Geometry: final body of the model. Coordinates: model frame, mm. A direction names the side the tool comes from. Give positions to 0.01 mm unless a question says otherwise; leave off trailing zeros. Loops run counter-clockwise (first coordinate to the right, second up) from the corner with the lowest first, then second, coordinate; pieces in that order, holes last. Notation, with made-up numbers: (8, 69.5) -> (41, 69.5) arc R15 cw to (41, 87.5) -> close; hole circle Ø6 at (19, 22). An arc over 180 degrees is marked (long way). Answer in a Markdown table with one row per item. Add a question column.
1) Section query A-A (y = -94). Return the cut outline in (x, z).
2) Line query: line 1 (Z direction, x = 0, y = -94); line 2 (Z direction, x = -99, y = -87); line 3 (X direction, y = -91, z = -73). Output: solid intervals per line, ascending. Write a range as from..to.
3) Section query D-D (z = -137). Return the cut outline in (x, y), plus the area to 3 significant figures.
4) First-contact query: P1, Ø2, axis at x = -19, z = -56, coming from the -Y side. Flat tip, straight axial feed; report the tip coordinate or a pass-through.
5) Section query C-C (z = 38.1). Return the cut outline in (x, y).
6) Draft query along X for faces 1 (the flat face through (-127, -60, -3)), 2 (the flat face through (-116.84, -68, -3)), 3 (the flat face through (-2, 0, -40)). Return one class per face: +X half, -X half, draft (parallel to the pull), parting line (faces both ways), or undercut.
7) Section query B-B (x = 0). Return the cut outline in (y, z), plus the area to 3 significant figures.
8) Access query for faces 4 (the flat face through (21.5, -127, 98.5)), 5 (the flat face through (-2, -68, -180.34)). Directions: +Z, -Z, +X, -X, +Y, -Y. A direction counts if a zero-diameter tool reaches every point of the face in a straight line with its end or side. Return the directions, or none.
```python
from build123d import *

# Parameters (mm, degrees)
F0_W     = 254
F0_H     = 381
F1_DEPTH = 127
F2_R     = 63.5
F3_DEPTH = 127.001
F4_T     = -10.16
F5_R     = 5.08


with BuildPart() as f1:
    # F0 (on Front) → F1 (new body)
    with BuildSketch(Plane.XZ):
        Rectangle(F0_W, F0_H)
    extrude(amount=F1_DEPTH)

    # F2 (on face) → F3 (cut, through all)
    with BuildSketch(Plane.XZ.offset(127)):
        with Locations((0, 38.1)):
            Circle(F2_R)
    extrude(amount=-F3_DEPTH, mode=Mode.SUBTRACT)

    # F4
    f4_openings = [f1.faces().sort_by_distance(p)[0] for p in [
        (0, -127, -185.92095),
    ]]
    offset(amount=F4_T, openings=f4_openings)

    # F5
    f5_edges = [f1.edges().sort_by_distance(p)[0] for p in [
        (-127, -127, 0),
        (0, -127, 190.5),
        (127, -127, 0),
        (0, -127, -190.5),
        (127, -63.5, -190.5),
        (127, -63.5, 190.5),
        (-127, -63.5, 190.5),
        (-127, -63.5, -190.5),
    ]]
    fillet(f5_edges, radius=F5_R)


solid = f1.part
```
Evaluation:
| question | item | result |
|---|---|---|
| 1 | outline | (-127, -185.42) arc R5.08 ccw to (-121.92, -190.5) -> (121.92, -190.5) arc R5.08 ccw to (127, -185.42) -> (127, 185.42) arc R5.08 ccw to (121.92, 190.5) -> (-121.92, 190.5) arc R5.08 ccw to (-127, 185.42) -> close; circle Ø147.32 at (0, 38.1); hole (-116.84, -180.34) -> (116.84, -180.34) -> (116.84, 180.34) -> (-116.84, 180.34) -> close; hole circle Ø127 at (0, 38.1) |
| 2 | line 1 | -190.5..-180.34, -35.56..-25.4, 101.6..111.76, 180.34..190.5 |
| 2 | line 2 | -190.5..-180.34, 180.34..190.5 |
| 2 | line 3 | -127..-116.84, 116.84..127 |
| 3 | outline | (-127, -121.92) arc R5.08 ccw to (-121.92, -127) -> (-116.84, -127) -> (-116.84, -10.16) -> (116.84, -10.16) -> (116.84, -127) -> (121.92, -127) arc R5.08 ccw to (127, -121.92) -> (127, 0) -> (-127, 0) -> close |
| 3 | area | 4,940 mm² |
| 4 | P1 | y = -10.16 |
| 5 | outline | (-127, -121.92) arc R5.08 ccw to (-121.92, -127) -> (-116.84, -127) -> (-116.84, -10.16) -> (-73.66, -10.16) -> (-73.66, -127) -> (-63.5, -127) -> (-63.5, 0) -> (-127, 0) -> close; (63.5, -127) -> (73.66, -127) -> (73.66, -10.16) -> (116.84, -10.16) -> (116.84, -127) -> (121.92, -127) arc R5.08 ccw to (127, -121.92) -> (127, 0) -> (63.5, 0) -> close |
| 6 | face 1 | -X half |
| 6 | face 2 | undercut |
| 6 | face 3 | draft |
| 7 | outline | (-127, -185.42) arc R5.08 ccw to (-121.92, -190.5) -> (0, -190.5) -> (0, -25.4) -> (-127, -25.4) -> (-127, -35.56) -> (-10.16, -35.56) -> (-10.16, -180.34) -> (-127, -180.34) -> close; (-127, 101.6) -> (0, 101.6) -> (0, 190.5) -> (-121.92, 190.5) arc R5.08 ccw to (-127, 185.42) -> (-127, 180.34) -> (-10.16, 180.34) -> (-10.16, 111.76) -> (-127, 111.76) -> close |
| 7 | area | 7,320 mm² |
| 8 | face 4 | +Z, -Z, +X, -X, -Y |
| 8 | face 5 | -Y |
